Work out the finished part from the listing and answer in its coordinate system (mm). Coordinates: 2 decimals unless noted, no trailing zeros. Order: outer loops, then holes, each group sorted by start corner. A loop starts at its lowest first (then second) coordinate and runs counter-clockwise, first axis right, second up. Notation, with made-up numbers: (24, 46.25) -> (46, 46.25) arc R7 ccw to (46, 50.25) -> close; hole circle Ø11 at (73, 83). An arc over 180 degrees is marked (long way). Answer as CSV lines item,"result". Start each with the question number.
Item 1: Section D-D (x = -3.5) is taken. Write down the section's boundary in (y, z), then the cut area to 3 significant figures.
Item 2: Section A-A (z = 0) is taken. Write down the section's boundary in (x, y).
Item 3: For a pull along Z with two mould halves and no side action, classify faces 1 (the face through (0.04, -0.54, -2.44)), 2 (the face through (0.07, -1.08, -4.88)) as pulls with the +Z half, pulls with the -Z half, needs draft (parallel to the pull), parting line crosses it, or undercut.
Item 4: Each of these flat-tipped pins is pushed along its axis until it touches: pin 1 Ø4 at (x, z) = (-2.5, -3.5) entering from -Y; pin 2 Ø2 at (x, y) = (0, -3) entering from +Z; pin 3 Ø5 at (x, z) = (-1, -3.5) entering from -Y. Where does it stop, or does it pass through?
Item 5: Section C-C (x = 1.25) is taken. Write down the section's boundary in (y, z), then the cut area to 3 significant figures.
Item 6: Straight lines are drawn through the part: L1, parallel to Z at x = 0.75, y = 0; L2, parallel to Z at x = 3.5, y = 0; L3, parallel to Y at x = 2, z = 2. For each, find the intervals that lie inside material, in ascending order.
```python
from build123d import *

# Parameters (mm, degrees)
F0_R     = 5
F1_DEPTH = 5
F2_R     = 2.5
F3_DEPTH = 25
F4_R     = 2


with BuildPart() as f1:
    # F0 (on Right) → F1 (new body, symmetric)
    with BuildSketch(Plane.YZ):
        Circle(F0_R)
    extrude(amount=F1_DEPTH, both=True)

    # F2 (on face) → F3 (cut)
    with BuildSketch(Plane.YZ.offset(5)):
        Circle(F2_R)
    extrude(amount=-F3_DEPTH, mode=Mode.SUBTRACT)

    # F4
    f4_edges = [f1.edges().sort_by_distance(p)[0] for p in [
        (5, -2.5, 0),
        (-5, -2.5, 0),
    ]]
    fillet(f4_edges, radius=F4_R)


solid = f1.part
```
Checked values:
1,outline,"circle Ø10 at (0, 0); hole circle Ø5.13 at (0, 0)"
1,area,"57.9 mm^2"
2,outline,"(-5, -5) -> (5, -5) -> (5, -4.5) arc R2 ccw to (3, -2.5) -> (-3, -2.5) arc R2 ccw to (-5, -4.5) -> close; (-5, 4.5) arc R2 ccw to (-3, 2.5) -> (3, 2.5) arc R2 ccw to (5, 4.5) -> (5, 5) -> (-5, 5) -> close"
3,face 1,"undercut"
3,face 2,"parting line crosses it"
4,pin 1,"stops at y = -4.77"
4,pin 2,"stops at z = 4.58"
4,pin 3,"stops at y = -4.9"
5,outline,"circle Ø10 at (0, 0); hole circle Ø5 at (0, 0)"
5,area,"58.9 mm^2"
6,L1,"z = -5 to -2.5, 2.5 to 5"
6,L2,"z = -5 to -2.56, 2.56 to 5"
6,L3,"y = -4.58 to -1.5, 1.5 to 4.58"
